CAD build for the part. Positions are in the model's coordinates, mm. Round coordinates to 2 decimals unless told otherwise and drop trailing zeros. Loops run counter-clockwise (first coordinate to the right, second up) from the corner with the lowest first, then second, coordinate; pieces in that order, holes last. Notation, with made-up numbers: M 7,84 L 33,84 A17 ccw 33,96 Z; hole C -6.5,74.25 d2. An arc over 180 degrees is marked long. One line per item, written item: value. Start each with the question number.
from build123d import *

# Parameters (mm, degrees)
F1_DEPTH = 37.5


with BuildPart() as f1:
    # F0 (on Front) → F1 (new body, symmetric)
    with BuildSketch(Plane.XZ):
        Polygon((99.613749, -334.373749), (-162.507823, -32.078042), (-203.583934, -150.890968), (58.537638, -453.186675), align=None)
        Polygon((202.636817, -453.186675), (99.613749, -334.373749), (58.537638, -453.186675), align=None)
    extrude(amount=F1_DEPTH, both=True)


solid = f1.part
(1) Probe L1, parallel to X at y = -20, z = -238; L2, parallel to Z at x = -151, y = -16.5; L3, parallel to X at y = 25, z = -79.5. List the from-to ranges inside material, lowest first.
(2) Slice it at B-B, the plane z = -116.5. List the corners of the cut face in (x, y), and give its area (3 significant figures).
(3) Slice it at C-C, the plane x = 125.5. List the corners of the cut face in (y, z).
(4) Slice it at A-A, the plane y = 29. List the corners of the cut face in (x, z), and give its area (3 significant figures).
(5) Flat gauge pins, fed straight in: P1, Ø5, axis at x = -111, y = 14.5, coming from the +Z side; P2, Ø10, axis at y = -7, z = -298.5, coming from the +X side; P3, Ø5, axis at x = 11, y = 15, coming from the +Z side. Where does each tip first touch, or does it go through?
Check result:
1. L1: x = -128.05 to 16.05
1. L2: z = -211.53 to -45.35
1. L3: x = -178.9 to -121.39
2. outline: M -191.69,-37.5 L -89.31,-37.5 L -89.31,37.5 L -191.69,37.5 Z
2. area: 7,680 mm^2
3. outline: M -37.5,-453.19 L 37.5,-453.19 L 37.5,-364.23 L -37.5,-364.23 Z
4. outline: M -203.58,-150.89 L 58.54,-453.19 L 202.64,-453.19 L -162.51,-32.08 Z
4. area: 52,100 mm^2
5. P1: stops at z = -88.6
5. P2: stops at x = 72.84
5. P3: stops at z = -229.3
